Autodesk Inventor part; units mm, degrees
ref_plane "YZ Plane" through (0, 0, 0) normal (1, 0, 0) x (0, 1, 0)
ref_plane "XZ Plane" through (0, 0, 0) normal (0, 1, 0) x (-1, 0, 0)
ref_plane "XY Plane" through (0, 0, 0) normal (0, 0, 1) x (1, 0, 0)
sketch "スケッチ1" plane through (0, 0, 0) normal (0, 0, 1) x (1, 0, 0)
  circle A0 centre (0, 0) radius 1.6
  circle A1 centre (0, 45) radius 11.05
  line L0 (0, 0) -> (0, 45) construction
  line L1 (0, 45) -> (38.9982, 362.6148) construction
  arc A2 (38.9982, 362.6148) -> (-16.4764, 170.4134) centre (231.3937, 202.9777) ccw
  line L2 (0, 45) -> (-6.5129, 94.574) construction
  arc A3 (-16.4764, 170.4134) -> (6.0935, 94.6273) centre (231.3937, 202.9777) ccw construction
  arc A4 (-14.6969, 42) -> (14.6249, 41.6667) centre (0, 45) ccw construction
  arc A5 (4.875, -1.1111) -> (-4.875, -1.1111) centre (0, 0) ccw construction
  line L3 (-14.7808, 42.3506) -> (-4.875, -1.1111)
  line L4 (14.6249, 41.6667) -> (4.875, -1.1111)
  line L5 (13.601, 51.3255) -> (-6.5129, 94.574)
  line L6 (-6.5129, 94.574) -> (-16.4764, 170.4134)
  arc A6 (38.9982, 362.6148) -> (27.4545, 372.193) centre (33.2263, 367.4039) ccw
  arc A7 (27.4545, 372.193) -> (-31.3486, 168.4596) centre (231.3937, 202.9777) ccw
  line L7 (-31.3486, 168.4596) -> (-14.7808, 42.3506)
  arc A8 (13.601, 51.3255) -> (-14.2261, 40.2443) centre (0, 45) ccw construction
  arc A9 (14.6249, 41.6667) -> (13.601, 51.3255) centre (0, 45) ccw
  arc A10 (-4.875, -1.1111) -> (4.875, -1.1111) centre (0, 0) ccw
  circle A11 centre (33.2263, 367.4039) radius 1.6
  arc A12 (41.0983, 369.7011) -> (-20.1506, 175.8768) centre (231.3937, 202.9777) ccw construction
  arc A13 (32.7138, 373.7709) -> (-17.6145, 121.4982) centre (231.3937, 202.9777) ccw construction
  circle A14 centre (11.9561, 328.899) radius 1.6
  circle A15 centre (-14.4042, 293.6829) radius 1.6
  circle A16 centre (-17.2387, 249.7852) radius 1.6
  circle A17 centre (-30.5608, 207.8618) radius 1.6
  circle A18 centre (-18.8107, 165.471) radius 1.6
  circle A19 centre (11.9561, 328.899) radius 3 construction
  circle A20 centre (-14.4042, 293.6829) radius 3 construction
  circle A21 centre (-17.6145, 121.4982) radius 1.6
  line L8 (-25.0506, 120.5212) -> (-17.6145, 121.4982) construction
  line L9 (-17.6145, 121.4982) -> (-10.1784, 122.4751) construction
  line L10 (33.2263, 367.4039) -> (11.9561, 328.899) construction
  line L11 (11.9561, 328.899) -> (-14.4042, 293.6829) construction
  line L12 (-14.4042, 293.6829) -> (-17.2387, 249.7852) construction
  line L13 (-17.2387, 249.7852) -> (-30.5608, 207.8618) construction
  line L14 (-30.5608, 207.8618) -> (-18.8107, 165.471) construction
  line L15 (-18.8107, 165.471) -> (-17.6145, 121.4982) construction
  dimension "d0" = 3.2
  dimension "d1" = 22.1
  dimension "d2" = 45
  dimension "d3" = 173
  dimension "d4" = 250
  dimension "d6" = 50
  dimension "d7" = 320
  dimension "d8" = 30
  dimension "d9" = 10
  dimension "d10" = 50
  dimension "d11" = 7.5
  dimension "d12" = 3.2
  dimension "d13" = 3.2
  dimension "d14" = 3.2
  dimension "d15" = 3.2
  dimension "d16" = 3.2
  dimension "d17" = 3.2
  dimension "d18" = 6
  dimension "d19" = 6
  dimension "d20" = 3.2
extrude "押し出し1" add sketch "スケッチ1" along normal blind 3
properties part number "ハンド" material "アセタール樹脂、黒"
Geometry check sheet. Reference: the model listing, model coordinates, mm. A direction names the side the tool comes from. Coordinates: 2 decimals unless noted, no trailing zeros. Order: outer loops, then holes, each group sorted by start corner. A loop starts at its lowest first (then second) coordinate and runs counter-clockwise, first axis right, second up.
Item 1: Tool access check on faces 1 (the flat face through (-11.425, 131.963, 1.479)), 2 (the cylindrical face through (37.89, 373.28, 1.48)). Record the directions out of +Z, -Z, +X, -X, +Y, -Y that give a thin tool (end or side, any length) a straight path to the whole face; none if there is none.
Item 2: Depth check by flat-ended pin: pin 1 (3.5 mm diameter, centred on x = -17.24, y = 249.79, fed in from -Z); pin 2 (1.5 mm diameter, centred on x = 22, z = 2.5, fed in from +Y). Enter the tip coordinate at first touch or a pass-through.
Item 3: Section check A-A (z = 2.1). Count the separate pieces of the cut face and the enclosed holes in it, plus the area to 3 significant figures.
Item 4: Section check C-C (y = 136.5). Enter the section's corners in (x, z).
Item 5: Scan lines: line 1 along X through (y, z) = (211, 2.25); line 2 along Y through (x, z) = (20.5, 0.8); line 3 along Y through (x, z) = (20, 1.4). Record each from-to range of solid material in increasing order.
Item 6: Mould release check, pull along Y, two halves, no side actions. Record for faces 3 (the flat face through (-23.18, 106.29, 1.48)), 4 (the cylindrical face through (-23.63, 275, 1.48)), 5 (the cylindrical face through (-9.197, 270.919, 1.479)): released by +Y, released by -Y, zero draft, split by the parting line, or undercut.
Item 7: Section check B-B (x = 20). Enter the section's corners in (y, z).
Check sheet entries:
1. face 1: +Z, -Z, +X
1. face 2: +Z, -Z
2. pin 1: stops at z = 0
2. pin 2: stops at y = 366.36
3. separate pieces: 1
3. enclosed holes: 9
3. area: 6,070 mm2
4. outline: (-27.15, 0) - (-12.02, 0) - (-12.02, 3) - (-27.15, 3) - close
5. line 1: x = -33.48 to -18.48
5. line 2: y = 337.23 to 363.44
5. line 3: y = 336.44 to 362.78
6. face 3: released by -Y
6. face 4: split by the parting line
6. face 5: undercut
7. outline: (336.44, 0) - (362.78, 0) - (362.78, 3) - (336.44, 3) - close
